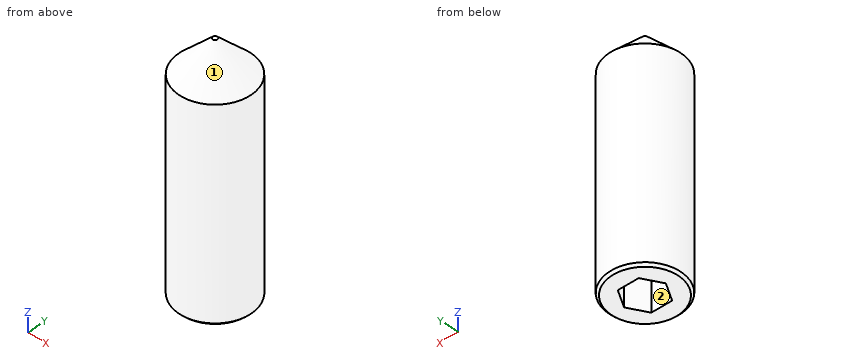
from build123d import *

# Parameters (mm, degrees)
SKETCH028_R     = 1.5
PAD013_DEPTH    = 10
CHAMFER003_SIZE = 1.4
POCKET014_DEPTH = 1.5
CHAMFER002_SIZE = 0.1


with BuildPart() as part:
    # Sketch028 → Pad013 (new body)
    with BuildSketch(Plane.XY):
        Circle(SKETCH028_R)
    extrude(amount=PAD013_DEPTH)

    # Chamfer003
    chamfer003_edges = [part.edges().sort_by_distance(p)[0] for p in [
        (-1.5, 0, 10),
    ]]
    chamfer(chamfer003_edges, length=CHAMFER003_SIZE)

    # Sketch027 → Pocket014 (cut)
    with BuildSketch(Plane.XY):
        Polygon((0.433013, -0.75), (0.866025, 0), (0.433013, 0.75), (-0.433013, 0.75), (-0.866025, 0), (-0.433013, -0.75), align=None)
    extrude(amount=POCKET014_DEPTH, mode=Mode.SUBTRACT)

    # Chamfer002
    chamfer002_edges = [part.edges().sort_by_distance(p)[0] for p in [
        (-1.5, 0, 0),
    ]]
    chamfer(chamfer002_edges, length=CHAMFER002_SIZE)


solid = part.part
The listing builds one solid part. Answer for the finished solid, in the listing's coordinates (mm). Face numbers are marked on the shaded views. A direction names the side the tool comes from. Give positions to 0.01 mm unless a question says otherwise; leave off trailing zeros. Loops run counter-clockwise (first coordinate to the right, second up) from the corner with the lowest first, then second, coordinate; pieces in that order, holes last. Notation, with made-up numbers: (-26.5, 5) - (15.5, 5) arc R24 cw to (15.5, 23) - close; hole circle Ø4 at (43, 51). An arc over 180 degrees is marked (long way). Use one line per item in the form item = value.
1. Find the intervals of material crossed by line 1 along Y through (x, z) = (-1.3, 3); line 2 along X through (y, z) = (-0.3, 1.25); line 3 along X through (y, z) = (1, 7.25), in increasing order. Write a range as [from, to].
Calculated:
line_1 = [-0.75, 0.75]
line_2 = [-1.47, -0.69], [0.69, 1.47]
line_3 = [-1.12, 1.12]
2. Which of the six approach directions +Z, -Z, +X, -X, +Y, -Y give full straight-line access (tool end or side, diameter ignored) to the marked faces 1 and 2?
Calculated:
face_1 = +Z
face_2 = -Z
3. Section A-A on z = 0.5 is taken. Give the vertices of the cut face in (x, y), then the cut area to 3 significant figures.
Calculated:
outline = circle Ø3 at (0, 0); hole (-0.87, 0) - (-0.43, -0.75) - (0.43, -0.75) - (0.87, 0) - (0.43, 0.75) - (-0.43, 0.75) - close
area = 5.12 mm^2
4. Section B-B on x = 0 is taken. Give the vertices of the cut face in (y, z).
Calculated:
outline = (-1.5, 0.1) - (-1.4, 0) - (-0.75, 0) - (-0.75, 1.5) - (0.75, 1.5) - (0.75, 0) - (1.4, 0) - (1.5, 0.1) - (1.5, 8.6) - (0.1, 10) - (-0.1, 10) - (-1.5, 8.6) - close
5. Section C-C on z = 6.25 is taken. Give the vertices of the cut face in (x, y), then the cut area to 3 significant figures.
Calculated:
outline = circle Ø3 at (0, 0)
area = 7.07 mm^2
